```python
from build123d import *

# Parameters (mm, degrees)
SKETCH1_W           = 38
SKETCH1_H           = 50
BOSS_EXTRUDE1_DEPTH = 1.7
SKETCH3_W           = 22.534452401
SKETCH3_H           = 28.525832834
BOSS_EXTRUDE2_DEPTH = 3
SKETCH4_W           = 0.314102564
SKETCH4_H           = 3.5
CUT_EXTRUDE2_DEPTH  = 0.3


with BuildPart() as part:
    # Sketch1 → Boss-Extrude1 (new body)
    with BuildSketch(Plane.XY):
        Rectangle(SKETCH1_W, SKETCH1_H)
    extrude(amount=BOSS_EXTRUDE1_DEPTH)

    # Sketch3 → Boss-Extrude2 (add)
    with BuildSketch(Plane.XY.offset(1.7)):
        with Locations((0.266789104, -0.871264125)):
            Rectangle(SKETCH3_W, SKETCH3_H)
    extrude(amount=BOSS_EXTRUDE2_DEPTH)

    # Sketch4 → Cut-Extrude2 (cut)
    with BuildSketch(Plane.XY.offset(4.7)):
        Polygon((-4.236247821, -0.83301235), (-3.91162843, -0.83301235), (-3.226632437, -3.399819241), (-2.207902469, -0.83301235), (-2.162329552, -0.83301235), (-1.162529873, -3.382291197), (-0.47402827, -0.83301235), (-0.152914488, -0.83301235), (-1.096624424, -4.33301235), (-1.141496219, -4.33301235), (-2.194581155, -1.656129338), (-3.260286283, -4.33301235), (-3.305158078, -4.33301235), align=None)
        with Locations((0.632341922, -2.58301235)):
            Rectangle(SKETCH4_W, SKETCH4_H)
        Polygon((1.686829102, -0.83301235), (3.391957307, -0.83301235), (3.391957307, -1.191986709), (2.000931666, -1.191986709), (2.000931666, -2.268909786), (3.391957307, -2.268909786), (3.391957307, -2.627884145), (2.000931666, -2.627884145), (2.000931666, -4.33301235), (1.686829102, -4.33301235), align=None)
        with Locations((4.177213717, -2.58301235)):
            Rectangle(SKETCH4_W, SKETCH4_H)
    extrude(amount=-CUT_EXTRUDE2_DEPTH, mode=Mode.SUBTRACT)


solid = part.part
```
CAD build for the part. Positions are in the model's coordinates, mm. A direction names the side the tool comes from. Round coordinates to 2 decimals unless told otherwise and drop trailing zeros. Loops run counter-clockwise (first coordinate to the right, second up) from the corner with the lowest first, then second, coordinate; pieces in that order, holes last. Notation, with made-up numbers: (89.5, 69.5) - (131.5, 69.5) arc R35 ccw to (131.5, 108.5) - close; hole circle Ø11 at (27.5, -2.5). An arc over 180 degrees is marked (long way). Return JSON: item names as keys, results as strings. Group by question number.
Q1. Band-saw the part on D-D on x = -16. Give the cut face in (y, z).
Q2. Two-plate mould, pull along X, no slides. Class faces 4 (the face through (-2.72, -2.98, 4.55)), 5 (the face through (0, 0, 0)), 6 (the face through (-11, -1, 3)), 7 (the face through (19, 0, 1)): +X half, -X half, draft (parallel to the pull), parting line (faces both ways), or undercut.
Q3. Band-saw the part on B-B on x = -9. Give the cut face in (y, z).
Q4. Drill centre lines: line 1 along Z through (x, y) = (-12, -8); line 2 along Y through (x, z) = (1, 4.35); line 3 along X through (y, z) = (10, 2.55). Where is each one in solid material? Low to high. Write a range as [from, to].
Q5. Tool access for faces 1 (the face through (0, 13.392, 3)), 2 (the face through (0, -15.134, 3)), 3 (the face through (11.534, -1, 3)): list every direction of +Z, -Z, +X, -X, +Y, -Y with a clear straight run to the whole face (end or side of a thin tool).
Q6. Band-saw the part on A-A on y = 12. Give the cut face in (x, z).
Q7. Flat gauge pins, fed straight in: pin 1 Ø1.5 at (y, z) = (-3.5, 3) entering from +X; pin 2 Ø2.5 at (x, z) = (-1.5, 4) entering from -Y. Where does each tip first touch, or does it go through?
Q8. Band-saw the part on C-C on z = 2.5. Give the cut face in (x, y).
Solutions:
{
 "1": {"outline": "(-25, 0) - (25, 0) - (25, 1.7) - (-25, 1.7) - close"},
 "2": {"face 4": "undercut", "face 5": "draft", "face 6": "-X half", "face 7": "+X half"},
 "3": {"outline": "(-25, 0) - (25, 0) - (25, 1.7) - (13.39, 1.7) - (13.39, 4.7) - (-15.13, 4.7) - (-15.13, 1.7) - (-25, 1.7) - close"},
 "4": {"line 1": "z = [0, 1.7]", "line 2": "y = [-15.13, 13.39]", "line 3": "x = [-11, 11.53]"},
 "5": {"face 1": "+Z, +X, -X, +Y", "face 2": "+Z, +X, -X, -Y", "face 3": "+Z, +X, +Y, -Y"},
 "6": {"outline": "(-19, 0) - (19, 0) - (19, 1.7) - (11.53, 1.7) - (11.53, 4.7) - (-11, 4.7) - (-11, 1.7) - (-19, 1.7) - close"},
 "7": {"pin 1": "stops at x = 11.53", "pin 2": "stops at y = -15.13"},
 "8": {"outline": "(-11, -15.13) - (11.53, -15.13) - (11.53, 13.39) - (-11, 13.39) - close"}
}
